from build123d import *

# Parameters (mm, degrees)
SKETCH_1_W             = 8
SKETCH_1_H             = 66
EXTRUDE_1_DEPTH        = 30
SKETCH_7_R             = 1.5
CUT_EXTRUDE_2_DEPTH    = 5
HOLE_WIZARD_M4_2_D     = 3.3
HOLE_WIZARD_M4_2_DEPTH = 10.1
HOLE_WIZARD_M4_2_TIP   = 0.991420021
SKETCH_10_R            = 1
CUT_EXTRUDE_4_DEPTH    = 5
HOLE_WIZARD_M3_1_D     = 2.5
HOLE_WIZARD_M3_1_DEPTH = 10.5
HOLE_WIZARD_M3_1_TIP   = 0.751075774
SKETCH_12_R            = 1
CUT_EXTRUDE_5_DEPTH    = 5
HOLE_WIZARD_M3_2_D     = 2.5
HOLE_WIZARD_M3_2_DEPTH = 18.5
HOLE_WIZARD_M3_2_TIP   = 0.751075774
SKETCH_14_W            = 8
SKETCH_14_H            = 7.5
CUT_EXTRUDE_6_DEPTH    = 30
SKETCH_15_R            = 6
CUT_EXTRUDE_7_DEPTH    = 84.024092889


with BuildPart() as part:
    # 草图1 → 凸台-拉伸1 (new body)
    with BuildSketch(Plane.XY):
        with Locations((14, -44)):
            Rectangle(SKETCH_1_W, SKETCH_1_H)
    extrude(amount=EXTRUDE_1_DEPTH)

    # 草图7 → 切除-拉伸2 (cut)
    with BuildSketch(Plane.ZY.offset(-10)):
        with Locations(Location((26.313708499, -44.686291501, 0), (0, 0, 270))):
            Circle(SKETCH_7_R)
        with Locations(Location((3.686291501, -44.686291501, 0), (0, 0, 90))):
            Circle(SKETCH_7_R)
        with Locations(Location((26.313708499, -67.313708499, 0), (0, 0, 90))):
            Circle(SKETCH_7_R)
        with Locations(Location((3.686291501, -67.313708499, 0), (0, 0, 270))):
            Circle(SKETCH_7_R)
    extrude(amount=-CUT_EXTRUDE_2_DEPTH, mode=Mode.SUBTRACT)

    # M4 螺纹孔2
    with Locations(Plane(origin=(18, -44.686291501, 3.686291501), x_dir=(0, 1, 0), z_dir=(1, 0, 0))):
        with Locations((0, 0), (-22.627416998, 0), (-22.627416998, 22.627416998), (0, 22.627416998)):
            Hole(HOLE_WIZARD_M4_2_D / 2, depth=HOLE_WIZARD_M4_2_DEPTH)
            with Locations((0, 0, -(HOLE_WIZARD_M4_2_DEPTH + HOLE_WIZARD_M4_2_TIP / 2))):  # 118° drill point
                Cone(0, HOLE_WIZARD_M4_2_D / 2, HOLE_WIZARD_M4_2_TIP, mode=Mode.SUBTRACT)

    # 草图10 → 切除-拉伸4 (cut)
    with BuildSketch(Plane(origin=(0, -11, 0), x_dir=(1, 0, 0), z_dir=(0, 1, 0))):
        with Locations(Location((14, -11.5, 0), (0, 0, 270))):
            Circle(SKETCH_10_R)
        with Locations(Location((14, -18.5, 0), (0, 0, 270))):
            Circle(SKETCH_10_R)
    extrude(amount=-CUT_EXTRUDE_4_DEPTH, mode=Mode.SUBTRACT)

    # M3 螺纹孔1
    with Locations(Plane(origin=(14, -11, 11.5), x_dir=(0, 0, 1), z_dir=(0, 1, 0))):
        with Locations((0, 0), (7, 0)):
            Hole(HOLE_WIZARD_M3_1_D / 2, depth=HOLE_WIZARD_M3_1_DEPTH)
            with Locations((0, 0, -(HOLE_WIZARD_M3_1_DEPTH + HOLE_WIZARD_M3_1_TIP / 2))):  # 118° drill point
                Cone(0, HOLE_WIZARD_M3_1_D / 2, HOLE_WIZARD_M3_1_TIP, mode=Mode.SUBTRACT)

    # 草图12 → 切除-拉伸5 (cut)
    with BuildSketch(Plane.XZ.offset(77)):
        with Locations(Location((14, 20, 0), (0, 0, 270))):
            Circle(SKETCH_12_R)
        with Locations(Location((14, 10, 0), (0, 0, 270))):
            Circle(SKETCH_12_R)
    extrude(amount=-CUT_EXTRUDE_5_DEPTH, mode=Mode.SUBTRACT)

    # M3 螺纹孔2
    with Locations(Plane(origin=(14, -77, 20), x_dir=(0, 0, -1), z_dir=(0, -1, 0))):
        with Locations((0, 0), (10, 0)):
            Hole(HOLE_WIZARD_M3_2_D / 2, depth=HOLE_WIZARD_M3_2_DEPTH)
            with Locations((0, 0, -(HOLE_WIZARD_M3_2_DEPTH + HOLE_WIZARD_M3_2_TIP / 2))):  # 118° drill point
                Cone(0, HOLE_WIZARD_M3_2_D / 2, HOLE_WIZARD_M3_2_TIP, mode=Mode.SUBTRACT)

    # 草图14 → 切除-拉伸6 (cut)
    with BuildSketch(Plane(origin=(0, -11, 0), x_dir=(1, 0, 0), z_dir=(0, 1, 0))):
        with Locations((14, -3.75)):
            Rectangle(SKETCH_14_W, SKETCH_14_H)
        with Locations((14, -26.25)):
            Rectangle(SKETCH_14_W, SKETCH_14_H)
    extrude(amount=-CUT_EXTRUDE_6_DEPTH, mode=Mode.SUBTRACT)

    # 草图15 → 切除-拉伸7 (cut, through all)
    with BuildSketch(Plane(origin=(18, 0, 0), x_dir=(0, 0, -1), z_dir=(1, 0, 0))):
        with Locations(Location((-15, -44, 0), (0, 0, 90))):
            Circle(SKETCH_15_R)
    extrude(amount=-CUT_EXTRUDE_7_DEPTH, mode=Mode.SUBTRACT)


solid = part.part
Here's how the part is built. I have some questions about the finished solid (model axes, mm). A direction names the side the tool comes from. Give positions to 0.01 mm unless a question says otherwise; leave off trailing zeros. Loops run counter-clockwise (first coordinate to the right, second up) from the corner with the lowest first, then second, coordinate; pieces in that order, holes last. Notation, with made-up numbers: (20, -16.5) -> (25, -16.5) arc R20 ccw to (25, -6.5) -> close; hole circle Ø11 at (12.25, -30.5). An arc over 180 degrees is marked (long way). One line per item, written item: value.
Q1. If I drill on line 1 along Z through (x, y) = (14, -13.75); line 2 along X through (y, z) = (-65.75, 10); line 3 along Z through (x, y) = (15, -60), over which ranges is the centre line in solid material (lowest first)?
Answers follow:
line 1: 7.5 to 10.25, 12.75 to 17.25, 19.75 to 22.5
line 2: 10 to 12.75, 15.25 to 18
line 3: 0 to 9.25, 10.75 to 19.25, 20.75 to 30
Q2. Suppose I cut it at C-C on z = 3. Please give me the cut outline in (x, y).
Answers follow:
outline: (10, -77) -> (18, -77) -> (18, -68.81) -> (10, -68.81) -> close; (10, -65.81) -> (18, -65.81) -> (18, -46.19) -> (10, -46.19) -> close; (10, -43.19) -> (18, -43.19) -> (18, -41) -> (10, -41) -> close
Q3. Suppose I cut it at A-A on y = -61.5. Please give me the cut outline in (x, z).
Answers follow:
outline: (10, 0) -> (18, 0) -> (18, 30) -> (10, 30) -> close; hole circle Ø2.5 at (14, 10); hole circle Ø2.5 at (14, 20)
Q4. I'm going to push flat-ended pins straight in: pin 1 Ø2.5 at (y, z) = (-67.31, 26.31) entering from -X; pin 2 Ø4 at (x, z) = (14.5, 27) entering from +Y; pin 3 Ø4 at (x, y) = (17, -20.5) entering from +Z; pin 4 Ø2 at (x, z) = (14, 11.5) entering from +Y. Where does each tip first touch, or does it pass through?
Answers follow:
pin 1: through
pin 2: y = -41
pin 3: z = 22.5
pin 4: y = -21.65
Q5. Suppose I cut it at D-D on x = 11. Please give me the cut outline in (y, z), then the cut area to 3 significant figures.
Answers follow:
outline: (-77, 0) -> (-41, 0) -> (-41, 7.5) -> (-11, 7.5) -> (-11, 22.5) -> (-41, 22.5) -> (-41, 30) -> (-77, 30) -> close; hole circle Ø3.3 at (-67.31, 3.69); hole circle Ø3.3 at (-67.31, 26.31); hole circle Ø12 at (-44, 15); hole circle Ø3.3 at (-44.69, 3.69); hole circle Ø3.3 at (-44.69, 26.31)
area: 1,380 mm^2
Q6. Suppose I cut it at B-B on z = 15. Please give me the cut outline in (x, y), then the cut area to 3 significant figures.
Answers follow:
outline: (10, -77) -> (18, -77) -> (18, -50) -> (10, -50) -> close; (10, -38) -> (18, -38) -> (18, -11) -> (10, -11) -> close
area: 432 mm^2
Q7. We'd pull the mould along Z, two halves only. Please class faces 5 (the face through (10, -52, 15)), 6 (the face through (14, -59, 0)), 7 (the face through (13.94, -46.21, 3.05)), 8 (the face through (15.054, -16.324, 17.828)): pulls with the +Z half, pulls with the -Z half, needs draft (parallel to the pull), parting line crosses it, or undercut.
Answers follow:
face 5: needs draft
face 6: pulls with the -Z half
face 7: undercut
face 8: undercut
Q8. On a 3-axis mill with a long thin cutter (end or side, diameter ignored), from which of +Z, -Z, +X, -X, +Y, -Y can I reach the whole of each face in a straight line? I mean faces 1 (the face through (14, -26, 22.5)), 2 (the face through (14.845, -67.62, 9.079)), 3 (the face through (14, -59, 30)), 4 (the face through (14, -26, 7.5)). Say none if no direction works.
Answers follow:
face 1: +Z, +X, -X, +Y
face 2: -Y
face 3: +Z, +X, -X, +Y, -Y
face 4: -Z, +X, -X, +Y
